Part model, mm, in its own coordinate system. A direction names the side the tool comes from. Round coordinates to 2 decimals unless told otherwise and drop trailing zeros. Order: outer loops, then holes, each group sorted by start corner. A loop starts at its lowest first (then second) coordinate and runs counter-clockwise, first axis right, second up. Notation, with made-up numbers: M 20.25,-30 L 57.25,-30 A10 ccw 57.25,-13 Z; hole C 59.25,38.25 d7. An arc over 180 degrees is marked long. One line per question, with ' | ' between items.
from build123d import *

# Parameters (mm, degrees)
SKETCH1_W           = 80.01
SKETCH1_H           = 200.025
BOSS_EXTRUDE1_DEPTH = 5.9944
SKETCH2_W           = 5.9944
SKETCH2_H           = 25.4
BOSS_EXTRUDE2_DEPTH = 5.9944
CUT_EXTRUDE1_DEPTH  = 6.9944


with BuildPart() as part:
    # Sketch1 → Boss-Extrude1 (new body)
    with BuildSketch(Plane.XY):
        with Locations((40.005, 100.0125)):
            Rectangle(SKETCH1_W, SKETCH1_H)
    extrude(amount=-BOSS_EXTRUDE1_DEPTH)

    # Sketch2 → Boss-Extrude2 (add)
    with BuildSketch(Plane.XY):
        with Locations((83.0072, 158.75)):
            Rectangle(SKETCH2_W, SKETCH2_H)
        with Locations((-2.9972, 158.75)):
            Rectangle(SKETCH2_W, SKETCH2_H)
        with Locations((-2.9972, 41.275)):
            Rectangle(SKETCH2_W, SKETCH2_H)
        with Locations((83.0072, 41.275)):
            Rectangle(SKETCH2_W, SKETCH2_H)
    extrude(amount=-BOSS_EXTRUDE2_DEPTH)

    # Sketch3 → Cut-Extrude1 (cut, through all)
    with BuildSketch(Plane.XY):
        Polygon((80.01, 195.453), (72.0852, 195.453), (72.0852, 197.6374), (69.0372, 197.6374), (69.0372, 195.453), (64.135, 195.453), (64.135, 191.897), (69.0372, 191.897), (69.0372, 189.7126), (72.0852, 189.7126), (72.0852, 191.897), (80.01, 191.897), align=None)
        Polygon((69.0372, 8.128), (64.135, 8.128), (64.135, 4.572), (69.0372, 4.572), (69.0372, 2.3876), (72.0852, 2.3876), (72.0852, 4.572), (80.01, 4.572), (80.01, 8.128), (72.0852, 8.128), (72.0852, 10.3124), (69.0372, 10.3124), align=None)
        Polygon((69.0372, 96.0501), (69.0372, 98.2345), (64.135, 98.2345), (64.135, 101.7905), (69.0372, 101.7905), (69.0372, 103.9749), (72.0852, 103.9749), (72.0852, 101.7905), (80.01, 101.7905), (80.01, 98.2345), (72.0852, 98.2345), (72.0852, 96.0501), align=None)
        Polygon((10.9728, 10.3124), (10.9728, 8.128), (15.875, 8.128), (15.875, 4.572), (10.9728, 4.572), (10.9728, 2.3876), (7.9248, 2.3876), (7.9248, 4.572), (0, 4.572), (0, 8.128), (7.9248, 8.128), (7.9248, 10.3124), align=None)
        Polygon((7.9248, 96.0501), (10.9728, 96.0501), (10.9728, 98.2345), (15.875, 98.2345), (15.875, 101.7905), (10.9728, 101.7905), (10.9728, 103.9749), (7.9248, 103.9749), (7.9248, 101.7905), (0, 101.7905), (0, 98.2345), (7.9248, 98.2345), align=None)
        Polygon((0, 195.453), (7.9248, 195.453), (7.9248, 197.6374), (10.9728, 197.6374), (10.9728, 195.453), (15.875, 195.453), (15.875, 191.897), (10.9728, 191.897), (10.9728, 189.7126), (7.9248, 189.7126), (7.9248, 191.897), (0, 191.897), align=None)
    extrude(amount=-CUT_EXTRUDE1_DEPTH, mode=Mode.SUBTRACT)


solid = part.part
1) Two-plate mould, pull along Y, no slides. Class faces 1 (the face through (76, 101.79, -3)), 2 (the face through (39, 101, 0)), 3 (the face through (39, 0, -3)): released by +Y, released by -Y, zero draft, split by the parting line, or undercut.
The answers:
face 1: undercut | face 2: zero draft | face 3: released by -Y
2) Probe line 1 (X direction, y = 190, z = -3.4); line 2 (Y direction, x = 10.5, z = -1.4) (3 decimals); line 3 (Y direction, x = 1, z = -1.55) (1 decimal). List the from-to ranges inside material, lowest first. Write a range as [from, to].
The answers:
line 1: x = [0, 7.92], [10.97, 69.04], [72.09, 80.01] | line 2: y = [0, 2.388], [10.312, 96.05], [103.975, 189.713], [197.637, 200.025] | line 3: y = [0, 4.6], [8.1, 98.2], [101.8, 191.9], [195.5, 200]
3) Saw through at B-B (y = 23.5). List the corners of the cut face in (x, z).
The answers:
outline: M 0,-5.99 L 80.01,-5.99 L 80.01,0 L 0,0 Z
4) Saw through at A-A (x = 74.5). List the corners of the cut face in (y, z) (1 decimal), plus the area to 3 significant figures.
The answers:
outline: M 0,-6 L 4.6,-6 L 4.6,0 L 0,0 Z; M 8.1,-6 L 98.2,-6 L 98.2,0 L 8.1,0 Z; M 101.8,-6 L 191.9,-6 L 191.9,0 L 101.8,0 Z; M 195.5,-6 L 200,-6 L 200,0 L 195.5,0 Z | area: 1,140 mm²
5) Drop flat-ended pins along their axis: pin 1 (1.5 mm diameter, centred on y = 128, z = -1, fed in from +X); pin 2 (3 mm diameter, centred on x = 84, z = -4, fed in from -Y) (3 decimals); pin 3 (0.7 mm diameter, centred on y = 97.5, z = -3, fed in from -X). Give the stop position or say it passes through.
The answers:
pin 1: stops at x = 80.01 | pin 2: stops at y = 28.575 | pin 3: stops at x = 0
6) Which spindle directions (+Z, -Z, +X, -X, +Y, -Y) get a long thin tool onto all of the face, cutting with end or side? Do faces 4 (the face through (4, 195.453, -3)), 5 (the face through (39, 101, -5.994)), 6 (the face through (-5.994, 41, -3)), 7 (the face through (67, 8.128, -3)), 8 (the face through (-3, 28.575, -3)). Say none if no direction does.
The answers:
face 4: +Z, -Z, -X | face 5: -Z, +X, -X, +Y, -Y | face 6: +Z, -Z, -X, +Y, -Y | face 7: +Z, -Z, +X | face 8: +Z, -Z, -X, -Y
